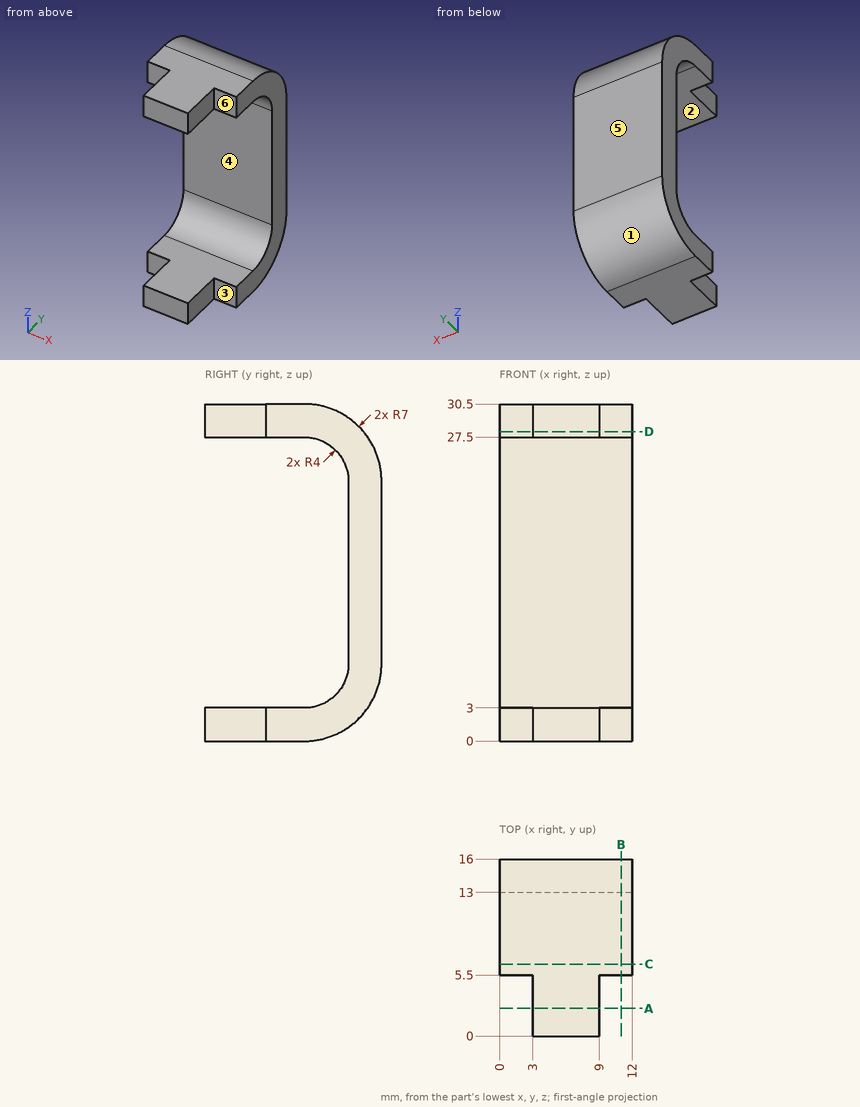
Here's the drawing with two shaded views (mm, measured from the low corner). I have some questions. A direction names the side the tool comes from. Coordinates: 2 decimals unless noted, no trailing zeros. Order: outer loops, then holes, each group sorted by start corner. A loop starts at its lowest first (then second) coordinate and runs counter-clockwise, first axis right, second up. Notation, with made-up numbers: (44, 71.25) - (83, 71.25) arc R10 ccw to (83, 79.25) - close; hole circle Ø6 at (49.25, 12.25). An arc over 180 degrees is marked (long way). Answer in a Markdown table with one row per item.
1. If I drill on line 1 along Z through (x, y) = (3.75, 3.5); line 2 along Y through (x, z) = (8.5, 16); line 3 along Z through (x, y) = (3.5, 12.25), over which ranges is the centre line in solid material (lowest first)?
Reply:
| item | result |
|---|---|
| line 1 | z = 0 to 3, 27.5 to 30.5 |
| line 2 | y = 13 to 16 |
| line 3 | z = 0.8 to 4.67, 25.83 to 29.7 |
2. If we mould it in two halves opening along Z, with no side actions, what happens to the marked faces 1, 2 and 3? For each: pulls with the +Z half, pulls with the -Z half, needs draft (parallel to the pull), parting line crosses it, or undercut.
Reply:
| item | result |
|---|---|
| face 1 | pulls with the -Z half |
| face 2 | undercut |
| face 3 | needs draft |
3. Suppose I cut it at D-D (z = 28). Please give me the cut outline in (x, y).
Reply:
| item | result |
|---|---|
| outline | (0, 5.5) - (3, 5.5) - (3, 0) - (9, 0) - (9, 5.5) - (12, 5.5) - (12, 14.36) - (0, 14.36) - close |
4. For the marked faces 4, 5 and 6, which set-ups out of +Z, -Z, +X, -X, +Y, -Y let a thin tool reach every point of the face, with its end or its side?
Reply:
| item | result |
|---|---|
| face 4 | +X, -X, -Y |
| face 5 | +Z, -Z, +X, -X, +Y |
| face 6 | +Z, -Z, +X, -Y |
5. Suppose I cut it at B-B (x = 11). Please give me the cut outline in (y, z).
Reply:
| item | result |
|---|---|
| outline | (5.5, 0) - (9, 0) arc R7 ccw to (16, 7) - (16, 23.5) arc R7 ccw to (9, 30.5) - (5.5, 30.5) - (5.5, 27.5) - (9, 27.5) arc R4 cw to (13, 23.5) - (13, 7) arc R4 cw to (9, 3) - (5.5, 3) - close |
6. Suppose I cut it at C-C (y = 6.5). Please give me the cut outline in (x, z), and give its area (3 significant figures).
Reply:
| item | result |
|---|---|
| outline | (0, 0) - (12, 0) - (12, 3) - (0, 3) - close; (0, 27.5) - (12, 27.5) - (12, 30.5) - (0, 30.5) - close |
| area | 72.0 mm^2 |
7. Suppose I cut it at A-A (y = 2.5). Please give me the cut outline in (x, z), and give its area (3 significant figures).
Reply:
| item | result |
|---|---|
| outline | (3, 0) - (9, 0) - (9, 3) - (3, 3) - close; (3, 27.5) - (9, 27.5) - (9, 30.5) - (3, 30.5) - close |
| area | 36.0 mm^2 |
8. For pin 1 (1.5 mm diameter, centred on y = 3.5, z = 2, fed in from +X); pin 2 (6 mm diameter, centred on x = 7, z = 15, fed in from -Y); pin 3 (5 mm diameter, centred on x = 8.5, z = 24.5, fed in from -Y); pin 4 (5 mm diameter, centred on y = 7, z = 7.5, fed in from +X), each with a flat end and sliding along its axis, tell me the tip position at first contact or that it passes through.
Reply:
| item | result |
|---|---|
| pin 1 | stops at x = 9 |
| pin 2 | stops at y = 13 |
| pin 3 | stops at y = 10.94 |
| pin 4 | passes through |
